```python
from build123d import *

# Parameters (mm, degrees)
BOSS_EXTRUDE1_DEPTH             = 70
CUT_EXTRUDE1_DEPTH              = 10
CUT_EXTRUDE2_DEPTH              = 10
M2_5_TAPPED_HOLE1_D             = 2.05
M2_5_TAPPED_HOLE1_DEPTH         = 10
M2_5_TAPPED_HOLE1_TIP           = 0.615882135
SKETCH8_W                       = 20
SKETCH8_H                       = 1.89069388
CUT_EXTRUDE3_DEPTH              = 14
M8_TAPPED_HOLE1_D               = 6.8
M8_TAPPED_HOLE1_DEPTH           = 6
M8_TAPPED_HOLE1_TIP             = 2.042926105
M3_TAPPED_HOLE1_D               = 2.5
M3_TAPPED_HOLE1_DEPTH           = 4
M3_TAPPED_HOLE1_TIP             = 0.751075774
M3_TAPPED_HOLE1_ON_FACE_2_D     = 2.5
M3_TAPPED_HOLE1_ON_FACE_2_DEPTH = 4
M3_TAPPED_HOLE1_ON_FACE_2_TIP   = 0.751075774
M2_TAPPED_HOLE1_D               = 1.6
BOSS_EXTRUDE2_DEPTH             = 50
FILLET1_R                       = 2


with BuildPart() as part:
    # Sketch1 → Boss-Extrude1 (new body)
    with BuildSketch(Plane.XY):
        Polygon((-29.059463918, 12.436342138), (-29.059463918, 0.436342138), (-57.250242541, 0.436342138), (-114.059463918, 0.436342138), (-114.059463918, 12.436342138), align=None)
        Polygon((-29.059463918, -0.303053562), (-57.250242541, -10.563657862), (-57.250242541, 0.436342138), (-29.059463918, 0.436342138), align=None)
    extrude(amount=BOSS_EXTRUDE1_DEPTH)

    # Sketch2 → Cut-Extrude1 (cut)
    with BuildSketch(Plane.XY.offset(70)):
        Polygon((-57.250242541, 0.436342138), (-29.059463918, 0.436342138), (-29.059463918, -0.303053562), (-57.250242541, -10.563657862), align=None)
    extrude(amount=-CUT_EXTRUDE1_DEPTH, mode=Mode.SUBTRACT)

    # Sketch3 → Cut-Extrude2 (cut)
    with BuildSketch(Plane(origin=(0, 0, 0), x_dir=(-1, 0, 0), z_dir=(0, 0, -1))):
        Polygon((57.250242541, 0.436342138), (57.250242541, -10.563657862), (29.059463918, -0.303053562), (29.059463918, 0.436342138), align=None)
    extrude(amount=-CUT_EXTRUDE2_DEPTH, mode=Mode.SUBTRACT)

    # M2.5 Tapped Hole1
    with Locations(Plane(origin=(-110.559463918, 12.436342138, 10.5), x_dir=(0, 0, 1), z_dir=(0, 1, 0))):
        with Locations((0, 0), (49, 0), (49, 58), (0, 58)):
            Hole(M2_5_TAPPED_HOLE1_D / 2, depth=M2_5_TAPPED_HOLE1_DEPTH)
            with Locations((0, 0, -(M2_5_TAPPED_HOLE1_DEPTH + M2_5_TAPPED_HOLE1_TIP / 2))):  # 118° drill point
                Cone(0, M2_5_TAPPED_HOLE1_D / 2, M2_5_TAPPED_HOLE1_TIP, mode=Mode.SUBTRACT)

    # Sketch8 → Cut-Extrude3 (cut)
    with BuildSketch(Plane.ZY.offset(114.059463918)):
        with Locations((35, 11.490995198)):
            Rectangle(SKETCH8_W, SKETCH8_H)
    extrude(amount=-CUT_EXTRUDE3_DEPTH, mode=Mode.SUBTRACT)

    # M8 Tapped Hole1
    with Locations(Plane(origin=(-34.697619642, -2.355174422, 35), x_dir=(-0.939692620786, -0.342020143326, 0), z_dir=(0.342020143326, -0.939692620786, 0))):
        with Locations((0, 0)):
            Hole(M8_TAPPED_HOLE1_D / 2, depth=M8_TAPPED_HOLE1_DEPTH)
            with Locations((0, 0, -(M8_TAPPED_HOLE1_DEPTH + M8_TAPPED_HOLE1_TIP / 2))):  # 118° drill point
                Cone(0, M8_TAPPED_HOLE1_D / 2, M8_TAPPED_HOLE1_TIP, mode=Mode.SUBTRACT)

    # M3 Tapped Hole1
    with Locations(Plane(origin=(-46.904584862, -6.798146413, 42.5), x_dir=(-0.939692620786, -0.342020143326, 0), z_dir=(0.342020143326, -0.939692620786, 0))):
        with Locations((0, 0)):
            Hole(M3_TAPPED_HOLE1_D / 2, depth=M3_TAPPED_HOLE1_DEPTH)
            with Locations((0, 0, -(M3_TAPPED_HOLE1_DEPTH + M3_TAPPED_HOLE1_TIP / 2))):  # 118° drill point
                Cone(0, M3_TAPPED_HOLE1_D / 2, M3_TAPPED_HOLE1_TIP, mode=Mode.SUBTRACT)

    # M3 Tapped Hole1 on face 2
    with Locations(Plane(origin=(-46.904584862, -6.798146413, 27.5), x_dir=(-0.939692711209, -0.342019894889, 0), z_dir=(0.342019894889, -0.939692711209, 0))):
        with Locations((0, 0)):
            Hole(M3_TAPPED_HOLE1_ON_FACE_2_D / 2, depth=M3_TAPPED_HOLE1_ON_FACE_2_DEPTH)
            with Locations((0, 0, -(M3_TAPPED_HOLE1_ON_FACE_2_DEPTH + M3_TAPPED_HOLE1_ON_FACE_2_TIP / 2))):  # 118° drill point
                Cone(0, M3_TAPPED_HOLE1_ON_FACE_2_D / 2, M3_TAPPED_HOLE1_ON_FACE_2_TIP, mode=Mode.SUBTRACT)

    # M2 Tapped Hole1 (through all)
    with Locations(Plane(origin=(-36.059463918, 12.436342138, 67.5), x_dir=(0, 0, 1), z_dir=(0, 1, 0))):
        with Locations((0, 0), (-65, 0), (-65, -56)):
            Hole(M2_TAPPED_HOLE1_D / 2)

    # Sketch17 → Boss-Extrude2 (add)
    with BuildSketch(Plane.XY.offset(60)):
        Polygon((-57.250242541, 0.436342138), (-77.407596349, 0.436342138), (-77.407596349, -17.900334649), (-57.250242541, -10.563657862), align=None)
    extrude(amount=-BOSS_EXTRUDE2_DEPTH)

    # Fillet1
    fillet1_edges = [part.edges().sort_by_distance(p)[0] for p in [
        (-77.407596349, -17.900334649, 35),
    ]]
    fillet(fillet1_edges, radius=FILLET1_R)


solid = part.part
```
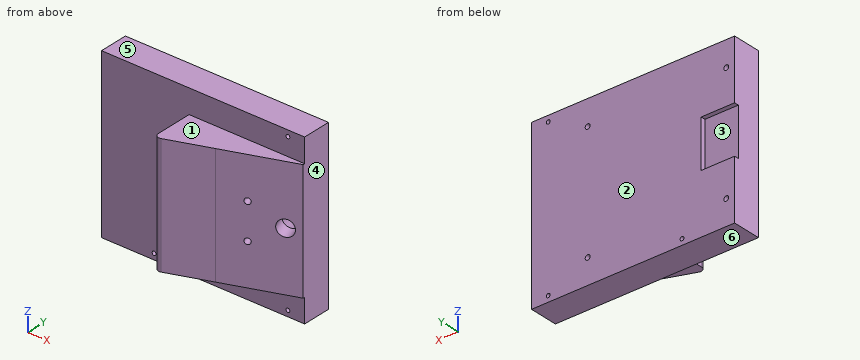
The listing builds one solid part. Answer for the finished solid, in the listing's coordinates (mm). Face numbers are marked on the shaded views. A direction names the side the tool comes from. Give positions to 0.01 mm unless a question says otherwise; leave off trailing zeros. Order: outer loops, then holes, each group sorted by start corner. A loop starts at its lowest first (then second) coordinate and runs counter-clockwise, first axis right, second up.
1) Find section A-A on z = 47. Write down the section's boundary in (x, y).
Reported:
outline: (-114.06, 0.44) - (-77.41, 0.44) - (-77.41, -15.04) arc R2 ccw to (-74.72, -16.92) - (-29.06, -0.3) - (-29.06, 12.44) - (-114.06, 12.44) - close
2) For the marked faces 1 and 2, determine the directions among +Z, -Z, +X, -X, +Y, -Y from which every point of the face is accessible in a straight line to the end or side of a thin tool.
Reported:
face 1: +Z, +X, -X, -Y
face 2: +Z, -Z, +X, -X, +Y
3) Find section D-D on z = 64. Write down the section's boundary in (x, y), then the cut area to 3 significant figures.
Reported:
outline: (-114.06, 0.44) - (-29.06, 0.44) - (-29.06, 12.44) - (-114.06, 12.44) - close
area: 1,020 mm2
4) Determine the mould class of the marked faces 3, 4, 5 and 6 for opening direction Z: pulls with the +Z half, pulls with the -Z half, needs draft (parallel to the pull), parting line crosses it, or undercut.
Reported:
face 3: undercut
face 4: needs draft
face 5: pulls with the +Z half
face 6: pulls with the -Z half
5) Consider line 1 along X through (y, z) = (8.25, 59.5); line 2 along X through (y, z) = (6.5, 67.5); line 3 along Y through (x, z) = (-51, 5). Determine where each line is inside the solid, lowest interval first.
Reported:
line 1: x = -114.06 to -111.58, -109.53 to -53.58, -51.53 to -29.06
line 2: x = -114.06 to -36.86, -35.26 to -29.06
line 3: y = 0.44 to 12.44
6) Given P1, Ø14, axis at x = -49, y = -9.5, coming from the -Z side; P2, Ø2.5, axis at x = -52.56, z = 59.5, coming from the -Y side; P3, Ø4.5, axis at y = -8.5, z = 41.5, coming from the -X side; P4, Ø10, axis at x = -82.5, y = -5, coming from the +Z side, each flat-ended and moving along its own axis, determine where each tip first touches the part or whether it passes through.
Reported:
P1: stops at z = 10
P2: stops at y = -9.31
P3: stops at x = -77.41
P4: passes through
7) Find section C-C on x = -88.5. Write down the section's boundary in (y, z).
Reported:
outline: (0.44, 0) - (12.44, 0) - (12.44, 70) - (0.44, 70) - close
8) Find section B-B on x = -55. Write down the section's boundary in (y, z), then the cut area to 3 significant figures.
Reported:
outline: (-9.74, 10) - (0.44, 10) - (0.44, 0) - (12.44, 0) - (12.44, 70) - (0.44, 70) - (0.44, 60) - (-9.74, 60) - close
area: 1,350 mm2
